The model under review builds one solid part; all positions refer to its coordinate system, in mm. A direction names the side the tool comes from. Round coordinates to 2 decimals unless told otherwise and drop trailing zeros. Loops run counter-clockwise (first coordinate to the right, second up) from the corner with the lowest first, then second, coordinate; pieces in that order, holes last. Notation, with made-up numbers: M 49.5,3 L 107.5,3 A26 ccw 107.5,23 Z; hole C -20.5,86 d9. An arc over 180 degrees is marked long. One line per question, with ' | ' between items.
from build123d import *

# Parameters (mm, degrees)
F0_W        = 10.6210811783
F0_H        = 127
F1_DEPTH    = 6.35
F2_DEPTH    = 6.35
F3_SIZE     = 5.334
F4_T2_ANGLE = 234.6452810907
F5_SIZE     = 5.588
F6_T1_DEPTH = 37.3754237446
F7_R        = 5.08
F8_R        = 5.08


# Not quite as in the source:
# - a fillet or chamfer that OpenCascade refuses, or shapes differently, is made with other operations: its cross-section is extruded or revolved along the edge and cut away or added
# - a feature names something its author has since deleted; it is built from what else it names


with BuildPart() as f1:
    # F0 (on Front) → F1 (new body)
    with BuildSketch(Plane.XZ):
        with BuildLine():
            ThreePointArc((-31.2650664442, 63.9850506011), (-26.8698078998, 60.1482815757), (-22.6583778858, 64.185972929))
            Line((-22.6583778858, 64.185972929), (-21.5300321579, 64.185972929))
            Line((-21.5300321579, 64.185972929), (-10.9089509796, 64.185972929))
            ThreePointArc((-10.9089509796, 64.185972929), (-1.1488196144, 60.4281603773), (3.5711703362, 51.0952608115))
            ThreePointArc((3.5711703362, 51.0952608115), (19.6335156732, 62.5824206191), (8.0880673261, 78.602920007))
            ThreePointArc((8.0880673261, 78.602920007), (0.2340476898, 70.6911078158), (-10.9089509796, 71.0316621421))
            Line((-10.9089509796, 71.0316621421), (-22.6583778858, 71.0316621421))
            ThreePointArc((-22.6583778858, 71.0316621421), (-25.8366796537, 75.4537471146), (-31.2650664442, 75.0189431538))
            Line((-31.2650664442, 75.0189431538), (-31.2650664442, 63.9850506011))
        make_face()
        with Locations((-16.2194915688, 0.685972929)):
            Rectangle(F0_W, F0_H)
    extrude(amount=F1_DEPTH)

    # F0 (on Front) → F2 (join)
    with BuildSketch(Plane.XZ):
        with BuildLine():
            ThreePointArc((-31.2650664442, 63.9850506011), (-26.8698078998, 60.1482815757), (-22.6583778858, 64.185972929))
            Line((-22.6583778858, 64.185972929), (-21.5300321579, 64.185972929))
            Line((-21.5300321579, 64.185972929), (-10.9089509796, 64.185972929))
            ThreePointArc((-10.9089509796, 64.185972929), (-1.1488196144, 60.4281603773), (3.5711703362, 51.0952608115))
            ThreePointArc((3.5711703362, 51.0952608115), (19.6335156732, 62.5824206191), (8.0880673261, 78.602920007))
            ThreePointArc((8.0880673261, 78.602920007), (0.2340476898, 70.6911078158), (-10.9089509796, 71.0316621421))
            Line((-10.9089509796, 71.0316621421), (-22.6583778858, 71.0316621421))
            ThreePointArc((-22.6583778858, 71.0316621421), (-25.8366796537, 75.4537471146), (-31.2650664442, 75.0189431538))
            Line((-31.2650664442, 75.0189431538), (-31.2650664442, 63.9850506011))
        make_face()
        with Locations((-16.2194915688, 0.685972929)):
            Rectangle(F0_W, F0_H)
    extrude(amount=-F2_DEPTH)

    # F3
    f3_edges = [f1.edges().sort_by_distance(p)[0] for p in [
        (19.633516, -6.35, 62.582421),
        (19.633516, 6.35, 62.582421),
    ]]
    chamfer(f3_edges, length=F3_SIZE)

    # F4: chamfer of 2.54 on 1 edges, made by hand

    # F4_s1 → F4_t2 (revolve, cut)
    with BuildSketch(Plane(origin=(-27.2674669531, 0, 20.2858371039), x_dir=(0, 1, 0), z_dir=(-0.8023210272, 0, 0.596892762))):
        Polygon((1.524, -41.5945799258), (-2.8120512242, -43.39063115), (-1.016, -41.5945799258), align=None)
    revolve(axis=Axis((5.8795952776, -1.016, 64.8408840236), (0, -1, 0)), revolution_arc=F4_T2_ANGLE, mode=Mode.SUBTRACT)

    # F5
    f5_edges = [f1.edges().sort_by_distance(p)[0] for p in [
        (-31.265066, 6.35, 69.501997),
        (-31.265066, -6.35, 69.501997),
    ]]
    chamfer(f5_edges, length=F5_SIZE)

    # F6: chamfer of 5.08 on 1 edges, made by hand

    # F6_s2 → F6_t1 (cut)
    with BuildSketch(Plane.XY.offset(50.8142850052)):
        Polygon((-31.2650664442, -4.318), (-27.6729639958, 4.3541024484), (-31.2650664442, 0.762), align=None)
    extrude(amount=F6_T1_DEPTH, mode=Mode.SUBTRACT)

    # F7
    f7_edges = [f1.edges().sort_by_distance(p)[0] for p in [
        (-10.908951, -6.35, 0.685973),
        (-10.908951, 6.35, 0.685973),
    ]]
    fillet(f7_edges, radius=F7_R)

    # F8
    f8_edges = [f1.edges().sort_by_distance(p)[0] for p in [
        (-21.530032, 6.35, 0.685973),
        (-21.530032, -6.35, 0.685973),
    ]]
    fillet(f8_edges, radius=F8_R)


solid = f1.part
1) Add section C-C on x = -13. State the section outline as (y, z) points.
Output values:
outline: M -6.35,64.03 L -5.38,64.03 L -5.38,-62.81 L 5.38,-62.81 L 5.38,64.03 L 6.35,64.03 L 6.35,71.03 L -6.35,71.03 Z
2) Add section B-B on y = -5. State the section outline as (x, z) points, then the cut area to 3 significant figures.
Output values:
outline: M -27.03,60.15 A4.32 ccw -22.66,64.19 L -19.9,64.19 L -19.9,-62.81 L -12.54,-62.81 L -12.54,64.09 A14.55 cw 2.4,55.51 A9.95 ccw long 5.86,74.79 A13.99 cw -10.91,71.03 L -22.66,71.03 A5.54 ccw -27.03,75.85 Z | area: 1,410 mm²
3) For line 1 (Z direction, x = -27.5, y = -3); line 2 (Z direction, x = -20, y = 0.75); line 3 (X direction, y = -1.75, z = -2), list the stretches that pass through material, from the lowest coordinate up.
Output values:
line 1: z = 60.18 to 75.93 | line 2: z = -62.81 to 71.03 | line 3: x = -21.51 to -10.93
4) Mouldability with a two-part tool opening along X and no side actions: class faces 4 (the flat face through (2, -6.35, 58)), 5 (the cylindrical face through (-24.631, -0.089, 60.835)), 6 (the flat face through (-27.982, -4.045, 68.168)) as +X half, -X half, draft (parallel to the pull), parting line (faces both ways), or undercut.
Output values:
face 4: draft | face 5: undercut | face 6: -X half
5) Machinability: for faces 1 (the flat face through (-28.966, 1.232, 67.975)), 2 (the flat face through (-17, 0, 71.032)), 3 (the flat face through (-22, 0, 64.186)), which of the approach directions +Z, -Z, +X, -X, +Y, -Y give a long, thin tool a straight path to every point of the face, cutting with its end or side? Answer none if there is none.
Output values:
face 1: +Z, -Z, -X, +Y | face 2: +Z, +Y, -Y | face 3: -Z
6) Add section A-A on z = -39. State the section outline as (x, y) points, then the cut area to 3 significant figures.
Output values:
outline: M -21.53,-1.27 A5.08 ccw -16.45,-6.35 L -15.99,-6.35 A5.08 ccw -10.91,-1.27 L -10.91,1.27 A5.08 ccw -15.99,6.35 L -16.45,6.35 A5.08 ccw -21.53,1.27 Z | area: 113 mm²
7) Add section D-D on y = 3. State the section outline as (x, z) points, then the cut area to 3 significant figures.
Output values:
outline: M -28.23,60.34 A4.32 ccw -22.66,64.19 L -21.23,64.19 L -21.23,-62.81 L -11.21,-62.81 L -11.21,64.18 A14.55 cw 3.2,53.19 A11.95 ccw long 7.19,76.72 A13.99 cw -10.91,71.03 L -22.66,71.03 A5.54 ccw -28.23,75.97 Z | area: 1,840 mm²
8) Insertion check: P1, Ø0.8, axis at y = 0, z = 26.5, coming from the -X side; P2, Ø3.5, axis at x = -18, y = -3, coming from the +Z side; P3, Ø1.3, axis at y = 0, z = 27.5, coming from the +X side. Each pin has a flat end and moves straight along its axis. Give the tip position at first contact, or say it passes through.
Output values:
P1: stops at x = -21.53 | P2: stops at z = 71.03 | P3: stops at x = -10.91
